The model under review builds one solid part; all positions refer to its coordinate system, in mm. Round coordinates to 2 decimals unless told otherwise and drop trailing zeros. Order: outer loops, then holes, each group sorted by start corner. A loop starts at its lowest first (then second) coordinate and runs counter-clockwise, first axis right, second up.
from build123d import *

# Parameters (mm, degrees)
SKETCH_1_W          = 138
SKETCH_1_H          = 88
SKETCH_1_R          = 1.6
EXTRUDE_1_DEPTH     = 4
FILLET_1_R          = 5
FILLET_2_R          = 5
SKETCH_2_R          = 4.5
CUT_EXTRUDE_1_DEPTH = 82.932899375
SKETCH_3_R          = 1.6
CUT_EXTRUDE_2_DEPTH = 82.932899375


with BuildPart() as part:
    # 草图1 → 凸台-拉伸1 (new body)
    with BuildSketch(Plane(origin=(0, 0, 0), x_dir=(1, 0, 0), z_dir=(0, 1, 0))):
        Rectangle(SKETCH_1_W, SKETCH_1_H)
        with Locations(Location((65, 40, 0), (0, 0, 270))):
            Circle(SKETCH_1_R, mode=Mode.SUBTRACT)
        with Locations(Location((65, -40, 0), (0, 0, 270))):
            Circle(SKETCH_1_R, mode=Mode.SUBTRACT)
        with Locations(Location((-65, -40, 0), (0, 0, 270))):
            Circle(SKETCH_1_R, mode=Mode.SUBTRACT)
        with Locations(Location((-65, 40, 0), (0, 0, 270))):
            Circle(SKETCH_1_R, mode=Mode.SUBTRACT)
        Polygon((-53.25, 38.769230769), (0, 6), (53.25, 38.769230769), align=None, mode=Mode.SUBTRACT)
        Polygon((53.25, -38.769230769), (0, -6), (-53.25, -38.769230769), align=None, mode=Mode.SUBTRACT)
        Polygon((-61.75, -34.307692308), (-6, 0), (-61.75, 34.307692308), align=None, mode=Mode.SUBTRACT)
        Polygon((61.75, -34.307692308), (6, 0), (61.75, 34.307692308), align=None, mode=Mode.SUBTRACT)
    extrude(amount=EXTRUDE_1_DEPTH)

    # 圆角1
    fillet_1_edges = [part.edges().sort_by_distance(p)[0] for p in [
        (0, 2, -6),
        (53.25, 2, -38.769230769),
        (-53.25, 2, -38.769230769),
        (0, 2, 6),
        (-53.25, 2, 38.769230769),
        (53.25, 2, 38.769230769),
        (-6, 2, 0),
        (-61.75, 2, -34.307692308),
        (-61.75, 2, 34.307692308),
        (61.75, 2, -34.307692308),
        (6, 2, 0),
        (61.75, 2, 34.307692308),
    ]]
    fillet(fillet_1_edges, radius=FILLET_1_R)

    # 圆角2
    fillet_2_edges = [part.edges().sort_by_distance(p)[0] for p in [
        (69, 2, 44),
        (-69, 2, 44),
        (-69, 2, -44),
        (69, 2, -44),
    ]]
    fillet(fillet_2_edges, radius=FILLET_2_R)

    # 草图2 → 切除-拉伸1 (cut, through all)
    with BuildSketch(Plane(origin=(0, 4, 0), x_dir=(1, 0, 0), z_dir=(0, 1, 0))):
        with Locations(Location((50.58680401, -36.855868382, 0), (0, 0, 270))):
            Circle(SKETCH_2_R)
        with Locations(Location((-50.58680401, -36.855868382, 0), (0, 0, 90))):
            Circle(SKETCH_2_R)
        with Locations(Location((-50.58680401, 36.855868382, 0), (0, 0, 270))):
            Circle(SKETCH_2_R)
        with Locations(Location((50.58680401, 36.855868382, 0), (0, 0, 90))):
            Circle(SKETCH_2_R)
    extrude(amount=-CUT_EXTRUDE_1_DEPTH, mode=Mode.SUBTRACT)

    # 草图3 → 切除-拉伸2 (cut, through all)
    with BuildSketch(Plane(origin=(0, 4, 0), x_dir=(1, 0, 0), z_dir=(0, 1, 0))):
        with Locations(Location((17.033166334, -10.481948513, 0), (0, 0, 270))):
            Circle(SKETCH_3_R)
        with Locations(Location((0, 0, 0), (0, 0, 270))):
            Circle(SKETCH_3_R)
    extrude(amount=-CUT_EXTRUDE_2_DEPTH, mode=Mode.SUBTRACT)


solid = part.part
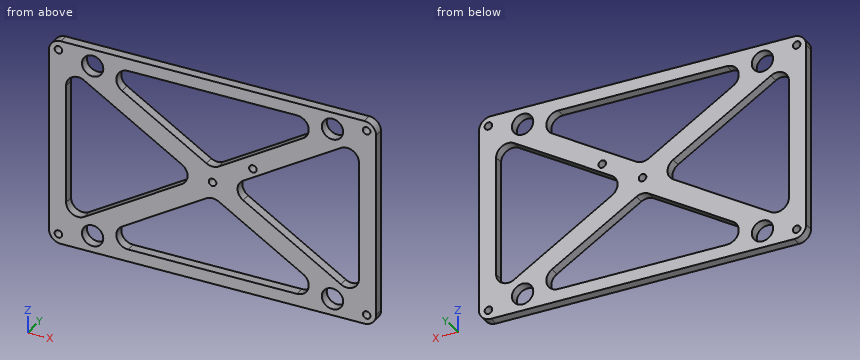
(1) We need section A-A (z = -22). Give the boundary of the cut face in (x, y), and give its area (3 significant figures).
(2) To check wall thickness, follow L1, parallel to X at y = 0.6, z = -22; L2, parallel to X at y = 2.2, z = -18.5; L3, parallel to Z at x = 65, y = 2.55. State the ranges of each line that lie inside material, in increasing order.
(3) We need section B-B (x = 42). Give the boundary of the cut face in (y, z).
(4) We need section D-D (x = -57). Give the boundary of the cut face in (y, z), and give its area (3 significant figures).
(5) We need section C-C (z = 0). Give the boundary of the cut face in (x, y).
Verdict:
1. outline: (-69, 0) - (-61.75, 0) - (-61.75, 4) - (-69, 4) - close; (-41.75, 0) - (-26, 0) - (-26, 4) - (-41.75, 4) - close; (26, 0) - (41.75, 0) - (41.75, 4) - (26, 4) - close; (61.75, 0) - (69, 0) - (69, 4) - (61.75, 4) - close
1. area: 184 mm2
2. L1: x = -69 to -61.75, -41.75 to -26, 26 to 41.75, 61.75 to 69
2. L2: x = -69 to -61.75, -36.06 to -20.31, 20.31 to 36.06, 61.75 to 69
2. L3: z = -43.9 to -41.6, -38.4 to 38.4, 41.6 to 43.9
3. outline: (0, -44) - (4, -44) - (4, -22.15) - (0, -22.15) - close; (0, 22.15) - (4, 22.15) - (4, 44) - (0, 44) - close
4. outline: (0, -44) - (4, -44) - (4, -30.35) - (0, -30.35) - close; (0, 30.35) - (4, 30.35) - (4, 44) - (0, 44) - close
4. area: 109 mm2
5. outline: (-69, 0) - (-61.75, 0) - (-61.75, 4) - (-69, 4) - close; (-10.54, 0) - (-1.6, 0) - (-1.6, 4) - (-10.54, 4) - close; (1.6, 0) - (10.54, 0) - (10.54, 4) - (1.6, 4) - close; (61.75, 0) - (69, 0) - (69, 4) - (61.75, 4) - close
